The model under review builds one solid part; all positions refer to its coordinate system, in mm. Face numbers are marked on the shaded views. A direction names the side the tool comes from. Give positions to 0.01 mm unless a question says otherwise; leave off trailing zeros. Loops run counter-clockwise (first coordinate to the right, second up) from the corner with the lowest first, then second, coordinate; pieces in that order, holes last. Notation, with made-up numbers: M 12,-19 L 18,-19 A21 ccw 18,-3 Z; hole C 6,-3.75 d8. An arc over 180 degrees is marked long. Return JSON: item names as keys, results as strings.
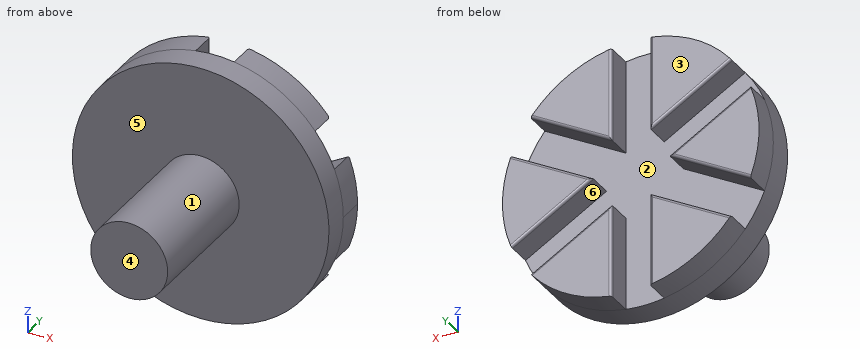
```python
from build123d import *

# Parameters (mm, degrees)
SKETCH1_R           = 127
BOSS_EXTRUDE1_DEPTH = 25.4
BOSS_EXTRUDE2_DEPTH = 25.4
SKETCH3_R           = 38.1
BOSS_EXTRUDE3_DEPTH = 127
FILLET1_R           = 2.54


with BuildPart() as part:
    # Sketch1 → Boss-Extrude1 (new body)
    with BuildSketch(Plane(origin=(0, 0, 0), x_dir=(1, 0, 0), z_dir=(0, 1, 0))):
        with Locations(Location((0, 0, 0), (0, 0, 90))):
            Circle(SKETCH1_R)
    extrude(amount=BOSS_EXTRUDE1_DEPTH)

    # Sketch2 → Boss-Extrude2 (add)
    with BuildSketch(Plane(origin=(0, 25.4, 0), x_dir=(1, 0, 0), z_dir=(0, 1, 0))):
        with BuildLine():
            Line((-118.25364463, -46.314960129), (-38.1, 0))
            Line((-38.1, 0), (-118.265853064, 46.283776846))
            ThreePointArc((-118.265853064, 46.283776846), (-126.999998896, -0.016743976), (-118.25364463, -46.314960129))
        make_face()
        with BuildLine():
            Line((-99.215853064, 79.27934473), (-19.05, 32.995567884))
            Line((-19.05, 32.995567884), (-19.05, 125.563121576))
            ThreePointArc((-19.05, 125.563121576), (-63.5, 109.985226281), (-99.215853064, 79.27934473))
        make_face()
        with BuildLine():
            Line((19.05, 125.563121576), (19.05, 32.995567884))
            Line((19.05, 32.995567884), (99.215853064, 79.27934473))
            ThreePointArc((99.215853064, 79.27934473), (63.5, 109.985226281), (19.05, 125.563121576))
        make_face()
        with BuildLine():
            Line((118.265853064, 46.283776846), (38.1, 0))
            Line((38.1, 0), (118.265853064, -46.283776846))
            ThreePointArc((118.265853064, -46.283776846), (124.79736243, -23.550336101), (127, 0))
            ThreePointArc((127, 0), (124.79736243, 23.550336101), (118.265853064, 46.283776846))
        make_face()
        with BuildLine():
            Line((99.215853064, -79.27934473), (19.05, -32.995567884))
            Line((19.05, -32.995567884), (19.05, -125.563121576))
            ThreePointArc((19.05, -125.563121576), (63.5, -109.985226281), (99.215853064, -79.27934473))
        make_face()
        with BuildLine():
            Line((-19.05, -125.563121576), (-19.05, -32.995567884))
            Line((-19.05, -32.995567884), (-99.194944867, -79.305503673))
            ThreePointArc((-99.194944867, -79.305503673), (-63.485498739, -109.993597313), (-19.05, -125.563121576))
        make_face()
    extrude(amount=BOSS_EXTRUDE2_DEPTH)

    # Sketch3 → Boss-Extrude3 (add)
    with BuildSketch(Plane.XZ):
        with Locations(Location((0, 0, 0), (0, 0, 270))):
            Circle(SKETCH3_R)
    extrude(amount=BOSS_EXTRUDE3_DEPTH)

    # Fillet1
    fillet1_edges = [part.edges().sort_by_distance(p)[0] for p in [
        (-59.132926532, 50.8, -56.137456307),
        (-19.05, 50.8, -79.27934473),
        (19.05, 50.8, -79.27934473),
        (59.132926532, 50.8, -56.137456307),
        (78.182926532, 50.8, -23.141888423),
        (78.182926532, 50.8, 23.141888423),
        (59.132926532, 50.8, 56.137456307),
        (19.05, 50.8, 79.27934473),
        (-19.05, 50.8, 79.27934473),
        (-59.122472434, 50.8, 56.150535779),
        (-78.176822315, 50.8, 23.157480064),
        (-78.182926532, 50.8, -23.141888423),
    ]]
    fillet(fillet1_edges, radius=FILLET1_R)


solid = part.part
```
1) Insertion check: pin 1 (2 mm diameter, centred on x = 39, y = 16.5, fed in from -Z); pin 2 (5 mm diameter, centred on y = -40.5, z = -4.5, fed in from +X); pin 3 (1.5 mm diameter, centred on x = 34.5, y = -36, fed in from +Z). Each pin has a flat end and moves straight along its axis. Give the tip position at first contact, or say it passes through.
From the geometry:
{"pin 1": "z = -121.18", "pin 2": "x = 38.05", "pin 3": "z = 17.68"}
2) Tool access review of the marked faces 4, 5 and 6: name each direction out of +Z, -Z, +X, -X, +Y, -Y from which nothing blocks a thin tool from reaching the whole face with its end or side.
From the geometry:
{"face 4": "+Z, -Z, +X, -X, -Y", "face 5": "-Y", "face 6": "+Y"}
3) Consider section B-B on y = -45. Write out the cut boundary in (x, z), then the cut area to 3 significant figures.
From the geometry:
{"outline": "C 0,0 d76.2", "area": "4,560 mm²"}
4) The part is to be moulded in two halves that separate along X. For the marked faces 1, 2 and 3, say which applies: released by +X, released by -X, zero draft, split by the parting line, or undercut.
From the geometry:
{"face 1": "split by the parting line", "face 2": "undercut", "face 3": "zero draft"}
5) Consider section A-A on x = 0. Write out the cut boundary in (y, z).
From the geometry:
{"outline": "M -127,-38.1 L 0,-38.1 L 0,-127 L 25.4,-127 L 25.4,127 L 0,127 L 0,38.1 L -127,38.1 Z"}
6) Wall thickness on L1, parallel to Z at x = 88.5, y = 31; L2, parallel to Y at x = -22, z = 93; L3, parallel to Y at x = 7, z = -30: over which ranges is each line inside the solid? List them lowest first. Write a range as from..to.
From the geometry:
{"L1": "-91.09..-73.09, -29.1..29.1, 73.09..91.09", "L2": "0..50.8", "L3": "-127..25.4"}
